Geometry: see drawing. Coordinates: mm, zero at the bounding-box minimum. A direction names the side the tool comes from. Coordinates: 2 decimals unless noted, no trailing zeros. Loops run counter-clockwise (first coordinate to the right, second up) from the corner with the lowest first, then second, coordinate; pieces in that order, holes last. Notation, with made-up numbers: (28, 39) -> (38, 39) arc R9 ccw to (38, 55) -> close; hole circle Ø5 at (14, 35). An arc over 180 degrees is marked (long way). One line per question, with ' | ' between items. Start each with the question number.
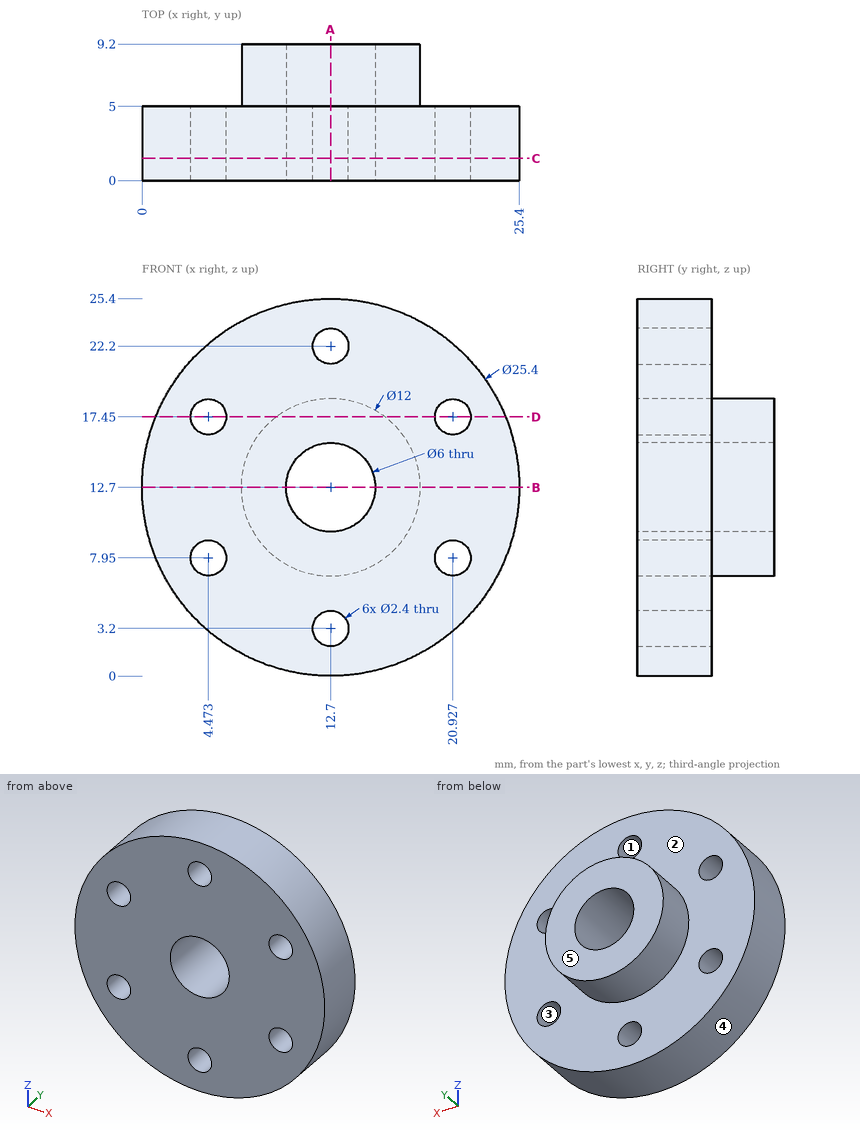
(1) Cut plane D-D, the plane z = 17.45. Return the cut outline in (x, y).
(2) Cut plane B-B, the plane z = 12.7. Return the cut outline in (x, y), and give its area (3 significant figures).
(3) Cut plane A-A, the plane x = 12.7. Return the cut outline in (y, z), and give its area (3 significant figures).
(4) Cut plane C-C, the plane y = 1.5. Return the cut outline in (x, z).
(5) Draft query along X for the marked faces 3, 4 and 5. Return one class per face: pulls with the +X half, pulls with the -X half, needs draft (parallel to the pull), parting line crosses it, or undercut.
(6) Ray query, L1, parallel to X at y = 3.85, z = 17.45; L2, parallel to X at y = 4, z = 18; L3, parallel to Z at x = 13.5, y = 2.5 (1 decimal). Return the intervals inside material, ascending.
(7) Access query for the marked faces 1 and 2. Directions: +Z, -Z, +X, -X, +Y, -Y. A direction counts if a zero-diameter tool reaches every point of the face in a straight line with its end or side. Return the directions, or none.
(8) Contact query for flat-ended pins moving along their axis: pin 1 Ø1.4 at (x, z) = (20.93, 7.95) entering from -Y; pin 2 Ø2 at (x, z) = (5.5, 6) entering from +Y; pin 3 Ø10 at (x, z) = (5, 20.5) entering from +Y; pin 4 Ø5 at (x, y) = (22.5, 5.5) entering from +Z. Output: stop coordinate, or through.
Here are the results:
1) outline: (0.92, 0) -> (3.27, 0) -> (3.27, 5) -> (0.92, 5) -> close; (5.67, 0) -> (19.73, 0) -> (19.73, 5) -> (16.37, 5) -> (16.37, 9.2) -> (9.03, 9.2) -> (9.03, 5) -> (5.67, 5) -> close; (22.13, 0) -> (24.48, 0) -> (24.48, 5) -> (22.13, 5) -> close
2) outline: (0, 0) -> (9.7, 0) -> (9.7, 9.2) -> (6.7, 9.2) -> (6.7, 5) -> (0, 5) -> close; (15.7, 0) -> (25.4, 0) -> (25.4, 5) -> (18.7, 5) -> (18.7, 9.2) -> (15.7, 9.2) -> close | area: 122 mm2
3) outline: (0, 0) -> (5, 0) -> (5, 2) -> (0, 2) -> close; (0, 4.4) -> (5, 4.4) -> (5, 6.7) -> (9.2, 6.7) -> (9.2, 9.7) -> (0, 9.7) -> close; (0, 15.7) -> (9.2, 15.7) -> (9.2, 18.7) -> (5, 18.7) -> (5, 21) -> (0, 21) -> close; (0, 23.4) -> (5, 23.4) -> (5, 25.4) -> (0, 25.4) -> close | area: 98.2 mm2
4) outline: circle Ø25.4 at (12.7, 12.7); hole circle Ø2.4 at (4.47, 7.95); hole circle Ø2.4 at (4.47, 17.45); hole circle Ø6 at (12.7, 12.7); hole circle Ø2.4 at (12.7, 3.2); hole circle Ø2.4 at (12.7, 22.2); hole circle Ø2.4 at (20.93, 7.95); hole circle Ø2.4 at (20.93, 17.45)
5) face 3: undercut | face 4: parting line crosses it | face 5: needs draft
6) L1: x = 0.92 to 3.27, 5.67 to 19.73, 22.13 to 24.48 | L2: x = 1.16 to 3.41, 5.54 to 19.86, 21.99 to 24.24 | L3: z = 0 to 2.3, 4.1 to 9.8, 15.6 to 21.3, 23.1 to 25.4
7) face 1: +Y, -Y | face 2: +Y
8) pin 1: passes through | pin 2: stops at y = 5 | pin 3: stops at y = 9.2 | pin 4: stops at z = 23.06
